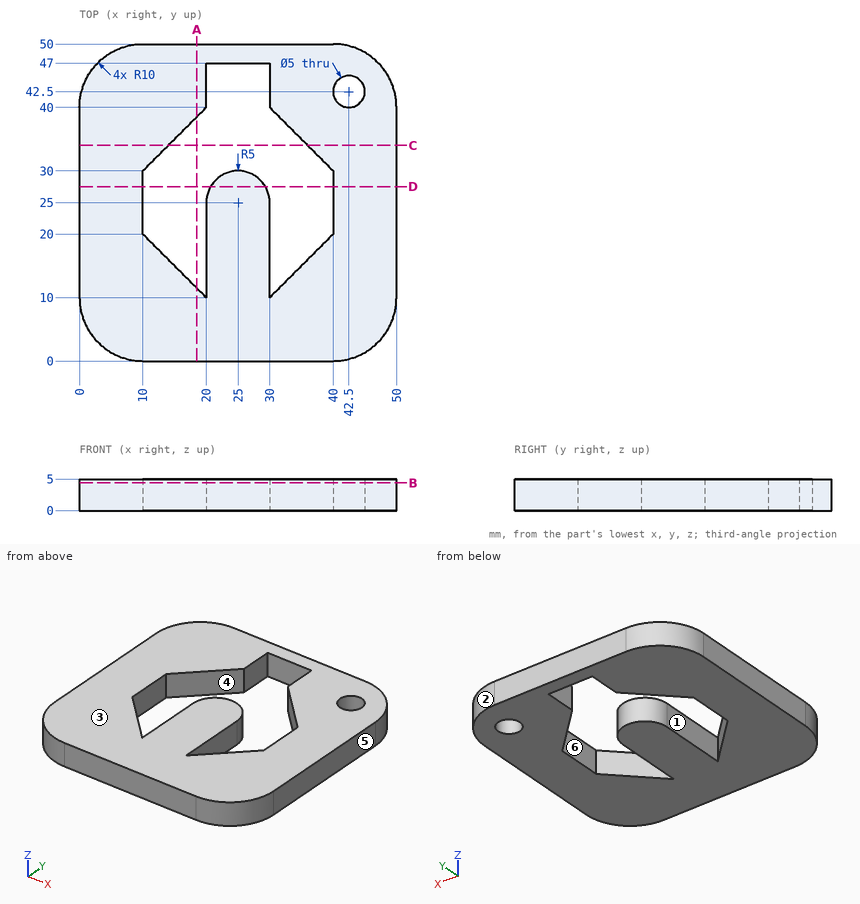
Can you work these out from the drawing? Everything is in mm from the part's minimum corner. A direction names the side the tool comes from. Give positions to 0.01 mm unless a question says otherwise; leave off trailing zeros. Loops run counter-clockwise (first coordinate to the right, second up) from the corner with the lowest first, then second, coordinate; pieces in that order, holes last. Notation, with made-up numbers: (29, 52.5) - (79, 52.5) arc R29 ccw to (79, 86.5) - close; hole circle Ø10 at (83, 25). An arc over 180 degrees is marked (long way). Answer as a JSON object with one key per item and string values.
Q1. Will these pins go through, and if not, where does the flat tip stop? P1, Ø3, axis at y = 6.5, z = 3, coming from the +X side; P2, Ø3, axis at x = 42.5, y = 42.5, coming from the +Z side.
Geometry says:
{"P1": "x = 49.8", "P2": "through"}
Q2. Imagine slicing it at B-B on z = 4.4. Write out the boundary of the cut face in (x, y).
Geometry says:
{"outline": "(0, 10) arc R10 ccw to (10, 0) - (40, 0) arc R10 ccw to (50, 10) - (50, 40) arc R10 ccw to (40, 50) - (10, 50) arc R10 ccw to (0, 40) - close; hole (10, 20) - (20, 10) - (20, 25) arc R5 cw to (30, 25) - (30, 10) - (40, 20) - (40, 30) - (30, 40) - (30, 47) - (20, 47) - (20, 40) - (10, 30) - close; hole circle Ø5 at (42.5, 42.5)"}
Q3. Which directions (+Z, -Z, +X, -X, +Y, -Y) give clear straight access to the entire face, cutting with the end or side of a thin tool? Please do the marked faces 1 and 2.
Geometry says:
{"face 1": "+Z, -Z", "face 2": "+Z, -Z, +X, +Y"}
Q4. Imagine slicing it at A-A on x = 18.5. Write out the boundary of the cut face in (y, z), plus the area to 3 significant figures.
Geometry says:
{"outline": "(0, 0) - (11.5, 0) - (11.5, 5) - (0, 5) - close; (38.5, 0) - (50, 0) - (50, 5) - (38.5, 5) - close", "area": "115 mm²"}
Q5. Imagine slicing it at D-D on y = 27.5. Write out the boundary of the cut face in (x, z).
Geometry says:
{"outline": "(0, 0) - (10, 0) - (10, 5) - (0, 5) - close; (20.67, 0) - (29.33, 0) - (29.33, 5) - (20.67, 5) - close; (40, 0) - (50, 0) - (50, 5) - (40, 5) - close"}
Q6. If we mould it in two halves opening along X, with no side actions, what happens to the marked faces 3, 4, 5 and 6? For each: pulls with the +X half, pulls with the -X half, needs draft (parallel to the pull), parting line crosses it, or undercut.
Geometry says:
{"face 3": "needs draft", "face 4": "undercut", "face 5": "pulls with the +X half", "face 6": "undercut"}
Q7. Imagine slicing it at C-C on y = 34. Write out the boundary of the cut face in (x, z).
Geometry says:
{"outline": "(0, 0) - (14, 0) - (14, 5) - (0, 5) - close; (36, 0) - (50, 0) - (50, 5) - (36, 5) - close"}
Q8. If I drill on L1, parallel to X at y = 25, z = 4.25; L2, parallel to X at y = 12, z = 1.4; L3, parallel to X at y = 32, z = 1.1, over which ranges is the centre line in solid material (lowest first)?
Geometry says:
{"L1": "0 to 10, 20 to 30, 40 to 50", "L2": "0 to 18, 20 to 30, 32 to 50", "L3": "0 to 12, 38 to 50"}
